```python
from build123d import *

# Parameters (mm, degrees)
SKETCH_2_R           = 4
EXTRUDE_1_DEPTH      = 35
EXTRUDE_2_DEPTH      = 4
EXTRUDE_2_DEPTH_BACK = 4
SKETCH_3_R           = 10.770329614
FILLET_3_R           = 1


with BuildPart() as part:
    # Sketch 1 → Revolve 1 (revolve)
    with BuildSketch(Plane.XY, mode=Mode.PRIVATE) as revolve_1_sk:
        Polygon((0, 0), (5, 0), (33, -22), (33, -42), (30, -42), (30, -60), (40, -60), (40, -180), (0, -180), align=None)
    revolve(revolve_1_sk.sketch.rotate(Axis((0, -180, 0), (0, 1, 0)), 90), axis=Axis((0, -180, 0), (0, 1, 0)))

    # Sketch 2 → Extrude 1 (add)
    with BuildSketch(Plane(origin=(0, 0, 0), x_dir=(0, 0, -1), z_dir=(1, 0, 0))):
        with Locations(Location((0, -51, 0), (0, 0, 180))):
            Circle(SKETCH_2_R)
    extrude(amount=EXTRUDE_1_DEPTH)

    # Sketch 3 → Extrude 2 (add, two sides: drawn at the far end of the back side and taken through both)
    with BuildSketch(Plane.XY.offset(-EXTRUDE_2_DEPTH_BACK)):
        with Locations((45, -51)):
            Circle(SKETCH_3_R)
    extrude(amount=EXTRUDE_2_DEPTH + EXTRUDE_2_DEPTH_BACK)

    # Fillet 3
    fillet_3_edges = [part.edges().sort_by_distance(p)[0] for p in [
        (29.732137496, -50.999999996, -4.000000004),
        (0, -60, 30),
        (0, -42, 30),
        (0, -42, 33),
        (0, -22, 33),
    ]]
    fillet(fillet_3_edges, radius=FILLET_3_R)


solid = part.part
```
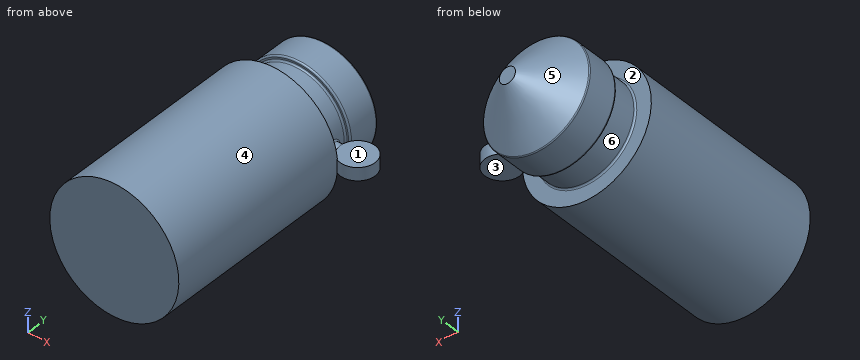
Geometry check sheet. Reference: the model listing, model coordinates, mm. Face numbers are marked on the shaded views. A direction names the side the tool comes from. Round coordinates to 2 decimals unless told otherwise and drop trailing zeros. Order: outer loops, then holes, each group sorted by start corner. A loop starts at its lowest first (then second) coordinate and runs counter-clockwise, first axis right, second up. Notation, with made-up numbers: (5, 66.5) -> (53, 66.5) arc R25 cw to (53, 100.5) -> close; hole circle Ø3 at (77, 77). An arc over 180 degrees is marked (long way). Return JSON: item names as keys, results as strings. Group by question number.
Q1. Section check B-B, the plane x = 45. Record the boundary of the cut face in (y, z).
Q2. Gauge pin test, flat ends, axial feed: pin 1 (1 mm diameter, centred on y = -98, z = -26.5, fed in from -X); pin 2 (12 mm diameter, centred on x = -17.5, y = -87.5, fed in from -Z); pin 3 (12 mm diameter, centred on y = -44.5, z = 4.5, fed in from -X). Record the tip position at first contact, or that the pin passes through.
Q3. Release check for a two-part mould opening along Y. For the marked faces 4, 5 and 6 record: released by +Y, released by -Y, zero draft, split by the parting line, or undercut.
Q4. Tool access check on the marked faces 1, 2 and 3. Record the directions out of +Z, -Z, +X, -X, +Y, -Y that give a thin tool (end or side, any length) a straight path to the whole face; none if there is none.
Q5. Material ranges on probe 1 along Y at (x, z) = (36.5, -12); probe 2 along Y at (x, z) = (-7.5, 31); probe 3 along Y at (x, z) = (2, 11), recorded low to high. Write a range as from..to.
Q6. Section check A-A, the plane y = -109. Record the boundary of the cut face in (x, z), plus the area to 3 significant figures.
Numbers:
{
 "1": {"outline": "(-61.77, -4) -> (-40.23, -4) -> (-40.23, 4) -> (-61.77, 4) -> close"},
 "2": {"pin 1": "x = -30.4", "pin 2": "z = -38.31", "pin 3": "x = -33"},
 "3": {"face 4": "zero draft", "face 5": "released by +Y", "face 6": "undercut"},
 "4": {"face 1": "+Z, +X, +Y", "face 2": "none", "face 3": "-Z, +X, +Y"},
 "5": {"probe 1": "-180..-60", "probe 2": "-180..-60, -42..-21.13", "probe 3": "-180..-4.86"},
 "6": {"outline": "circle Ø80 at (0, 0)", "area": "5,030 mm^2"}
}
